```python
from build123d import *

# Parameters (mm, degrees)
SKETCH001_R         = 1.1
SKETCH001_W         = 13
SKETCH001_H         = 24
PAD_DEPTH           = 5
HOLE_D              = 2.4
HOLE_CBORE_D        = 4.3
HOLE_CBORE_DEPTH    = 1.6
SKETCH003_W         = 10
SKETCH003_H         = 20
PAD001_DEPTH        = 3
PAD002_DEPTH        = 3
SKETCH005_R         = 2.5
PAD003_DEPTH        = 3
SKETCH006_R         = 2.5
SKETCH006_R_2       = 2
POCKET_DEPTH        = 2
CHAMFER_SIZE        = 0.49
FILLET_R            = 0.5
HOLE001_D           = 2.4
HOLE001_DEPTH       = 25
HOLE001_CBORE_D     = 4.3
HOLE001_CBORE_DEPTH = 1.6


with BuildPart() as part:
    # Sketch001 → Pad (new body)
    with BuildSketch(Plane.XZ):
        Polygon((48.504088, 55), (-26.495912, 55), (-38.495912, 7.5), (-32.166242, -16.5), (-37.166242, -16.5), (-37.166242, -18.5), (-32.166242, -18.5), (-26.495912, -40), (48.504088, -40), (48.504088, -42.5), (98.504088, -42.5), (98.504088, 7.5), (48.504088, 7.5), align=None)
        with Locations((87.004088, -7.5)):
            Circle(SKETCH001_R, mode=Mode.SUBTRACT)
        with Locations((87.004141, -35.5)):
            Circle(SKETCH001_R, mode=Mode.SUBTRACT)
        Polygon((-22.334011, 49), (-32.818222, 7.5), (-21.873167, -34), (-0.995912, -1), (42.504088, -1), (42.504088, 7.5), (42.504088, 16), (-0.995912, 16), align=None, mode=Mode.SUBTRACT)
        Polygon((42.504088, 49), (-15.188963, 49), (2.269482, 22), (42.504088, 22), align=None, mode=Mode.SUBTRACT)
        with Locations((87.004088, -21.5)):
            Rectangle(SKETCH001_W, SKETCH001_H, mode=Mode.SUBTRACT)
    extrude(amount=PAD_DEPTH)

    # Hole (through all)
    with Locations(Plane.XZ.offset(5)):
        with Locations((-13.5, 52.391686), (11.75, 52.391686), (37, 52.391686), (-13.5, -37.391686), (11.75, -37.391686), (37, -37.391686)):
            CounterBoreHole(HOLE_D / 2, HOLE_CBORE_D / 2, HOLE_CBORE_DEPTH)

    # Sketch003 → Pad001 (join)
    with BuildSketch(Plane.XZ):
        with Locations((-23.495912, 53.5)):
            Rectangle(SKETCH003_W, SKETCH003_H)
        with Locations((47.504088, 53.5)):
            Rectangle(SKETCH003_W, SKETCH003_H)
        with Locations((-23.495912, -38.5)):
            Rectangle(SKETCH003_W, SKETCH003_H)
        with Locations((47.504088, -38.5)):
            Rectangle(SKETCH003_W, SKETCH003_H)
    extrude(amount=-PAD001_DEPTH)

    # Sketch004 (on Face6 of Pad001) → Pad002 (join)
    with BuildSketch(Plane.XZ.offset(5)):
        with BuildLine():
            ThreePointArc((-3.495912, -9), (-4.995912, -10.5), (-3.495912, -12))
            Line((-3.495912, -12), (56.504088, -12))
            ThreePointArc((56.504088, -12), (58.004088, -10.5), (56.504088, -9))
            Line((-3.495912, -9), (56.504088, -9))
        make_face()
        with BuildLine():
            ThreePointArc((-3.495912, -23), (-4.995912, -24.5), (-3.495912, -26))
            Line((-3.495912, -26), (56.504088, -26))
            ThreePointArc((56.504088, -26), (58.004088, -24.5), (56.504088, -23))
            Line((-3.495912, -23), (56.504088, -23))
        make_face()
    extrude(amount=PAD002_DEPTH)

    # Sketch005 → Pad003 (join)
    with BuildSketch(Plane(origin=(0, 0, 0), x_dir=(1, 0, 0), z_dir=(0, 1, 0))):
        with Locations((-30.382342, 12.5)):
            Circle(SKETCH005_R)
        with Locations((-33.019704, 2.5)):
            Circle(SKETCH005_R)
        with Locations((-35.657067, -7.5)):
            Circle(SKETCH005_R)
        with Locations((-33.130751, -17.5)):
            Circle(SKETCH005_R)
        with Locations((-30.604435, -27.5)):
            Circle(SKETCH005_R)
        with Locations((-28.078119, -37.5)):
            Circle(SKETCH005_R)
    extrude(amount=PAD003_DEPTH)

    # Sketch006 → Pocket (cut)
    with BuildSketch(Plane(origin=(0, 0, 0), x_dir=(1, 0, 0), z_dir=(0, 1, 0))):
        with Locations((-30.382342, 12.5)):
            Circle(SKETCH006_R)
        with Locations((-30.382342, 12.5)):
            Circle(SKETCH006_R_2, mode=Mode.SUBTRACT)
        with Locations((-33.019704, 2.5)):
            Circle(SKETCH006_R)
        with Locations((-33.019704, 2.5)):
            Circle(SKETCH006_R_2, mode=Mode.SUBTRACT)
        with Locations((-35.657067, -7.5)):
            Circle(SKETCH006_R)
        with Locations((-35.657067, -7.5)):
            Circle(SKETCH006_R_2, mode=Mode.SUBTRACT)
        with Locations((-33.130751, -17.5)):
            Circle(SKETCH006_R)
        with Locations((-33.130751, -17.5)):
            Circle(SKETCH006_R_2, mode=Mode.SUBTRACT)
        with Locations((-30.604435, -27.5)):
            Circle(SKETCH006_R)
        with Locations((-30.604435, -27.5)):
            Circle(SKETCH006_R_2, mode=Mode.SUBTRACT)
        with Locations((-28.078119, -37.5)):
            Circle(SKETCH006_R)
        with Locations((-28.078119, -37.5)):
            Circle(SKETCH006_R_2, mode=Mode.SUBTRACT)
    extrude(amount=POCKET_DEPTH, mode=Mode.SUBTRACT)

    # Chamfer
    chamfer_edges = [part.edges().sort_by_distance(p)[0] for p in [
        (-30.078119, 0, 37.5),
        (-32.604435, 0, 27.5),
        (-35.130751, 0, 17.5),
        (-37.657067, 0, 7.5),
        (-35.019704, 0, -2.5),
        (-32.382342, 0, -12.5),
    ]]
    chamfer(chamfer_edges, length=CHAMFER_SIZE)

    # Fillet
    fillet_edges = [part.edges().sort_by_distance(p)[0] for p in [
        (-4.995912, -8, -24.5),
        (26.504088, -8, -26),
        (58.004088, -8, -24.5),
        (26.504088, -8, -23),
        (-4.995912, -8, -10.5),
        (26.504088, -8, -12),
        (58.004088, -8, -10.5),
        (26.504088, -8, -9),
    ]]
    fillet(fillet_edges, radius=FILLET_R)

    # Hole001
    with Locations(Plane(origin=(0, 0, 0), x_dir=(1, 0, 0), z_dir=(0, 1, 0))):
        with Locations((-10.495912, 26), (64.504088, 26)):
            CounterBoreHole(HOLE001_D / 2, HOLE001_CBORE_D / 2, HOLE001_CBORE_DEPTH, depth=HOLE001_DEPTH)


solid = part.part
```
Work out the finished part from the listing and answer in its coordinate system (mm). A direction names the side the tool comes from. Give positions to 0.01 mm unless a question says otherwise; leave off trailing zeros. Order: outer loops, then holes, each group sorted by start corner. A loop starts at its lowest first (then second) coordinate and runs counter-clockwise, first axis right, second up. Notation, with made-up numbers: (-18, -38.75) -> (39, -38.75) arc R26 ccw to (39, -9.75) -> close; hole circle Ø11 at (84, 7). An arc over 180 degrees is marked (long way). Answer as CSV lines item,"result". Start each with the question number.
(1) Section B-B, the plane z = -2.5 is taken. Write down the section's boundary in (x, y), plus the area to 3 significant figures.
(2) For a pull along Z with two mould halves and no side action, classify faces 5 (the flat face through (52.504, 1, 53)), 6 (the flat face through (-11.516, -2.465, 32.269)), 7 (the flat face through (-32.412, -2.465, 31.582)) as released by +Z, released by -Z, zero draft, split by the parting line, or undercut.
(3) Which of the six approach directions +Z, -Z, +X, -X, +Y, -Y give full straight-line access (tool end or side, diameter ignored) to faces 1 (the flat face through (-9, -1.6, -26)), 2 (the cylindrical face through (-34.605, 1.234, 16.148)), 3 (the flat face through (-28.496, 1, 53)), 4 (the flat face through (-18.496, 1, 53))?
(4) Section A-A, the plane x = 82 is taken. Write down the section's boundary in (y, z), plus the area to 3 significant figures.
(5) Section C-C, the plane z = 37.5 is taken. Write down the section's boundary in (x, y), plus the area to 3 significant figures.
(6) Each of these flat-tipped pins is pushed along its axis until it touches: pin 1 Ø1.5 at (y, z) = (2, 56) entering from -X; pin 2 Ø6 at (y, z) = (0, -34.5) entering from -X; pin 3 Ø1.4 at (x, z) = (64.5, -26) entering from +Y; pin 4 Ø3 at (y, z) = (0.5, 27.5) entering from +X. Where does it stop, or does it pass through?
(7) Consider line 1 along Z through (x, y) = (40.5, -0.75); line 2 along Z through (x, y) = (11.75, -2.65); line 3 along Z through (x, y) = (37, -4). Determine where each line is inside the solid, lowest interval first.
Entries:
1,outline,"(-35.86, -5) -> (-30.18, -5) -> (-30.18, 0) -> (-30.53, 0) -> (-31.02, 0.49) -> (-31.02, 2) -> (-30.52, 2) -> (-30.52, 3) -> (-35.52, 3) -> (-35.52, 2) -> (-35.02, 2) -> (-35.02, 0.49) -> (-35.51, 0) -> (-35.86, 0) -> close; (-1.94, -5) -> (98.5, -5) -> (98.5, 0) -> (-1.94, 0) -> close"
1,area,"544 mm²"
2,face 5,"zero draft"
2,face 6,"undercut"
2,face 7,"released by +Z"
3,face 1,"+Y"
3,face 2,"none"
3,face 3,"+Z, -X, +Y"
3,face 4,"+Z, -Z, +Y"
4,outline,"(-5, -42.5) -> (0, -42.5) -> (0, -33.5) -> (-5, -33.5) -> close; (-5, -9.5) -> (0, -9.5) -> (0, 7.5) -> (-5, 7.5) -> close"
4,area,"130 mm²"
5,outline,"(-30.92, -5) -> (-25.24, -5) -> (-25.24, 0) -> (-25.59, 0) -> (-26.08, 0.49) -> (-26.08, 2) -> (-25.58, 2) -> (-25.58, 3) -> (-30.58, 3) -> (-30.58, 2) -> (-30.08, 2) -> (-30.08, 0.49) -> (-30.57, 0) -> (-30.92, 0) -> close; (-14.9, -5) -> (-7.75, -5) -> (-7.75, 0) -> (-14.9, 0) -> close; (42.5, -5) -> (48.5, -5) -> (48.5, 0) -> (42.5, 0) -> close"
5,area,"107 mm²"
6,pin 1,"x = -28.5"
6,pin 2,"x = -28.74"
6,pin 3,"through"
6,pin 4,"x = 48.5"
7,line 1,"-40 to -1, 16 to 22, 49 to 55"
7,line 2,"-40 to -38.59, -36.19 to -1, 16 to 22, 49 to 51.19, 53.59 to 55"
7,line 3,"-40 to -39.54, -35.24 to -1, 16 to 22, 49 to 50.24, 54.54 to 55"
